```python
from build123d import *

# Parameters (mm, degrees)
SKETCH_1_W          = 10
SKETCH_1_H          = 10
SKETCH_1_W_2        = 8
SKETCH_1_H_2        = 8
EXTRUDE_1_DEPTH     = 40
SKETCH_2_R          = 1.6
CUT_EXTRUDE_1_DEPTH = 408.37168574
SKETCH_3_R          = 1.6
CUT_EXTRUDE_2_DEPTH = 10


with BuildPart() as part:
    # ｽｹｯﾁ1 → ﾎﾞｽ - 押し出し1 (new body)
    with BuildSketch(Plane.XY):
        Rectangle(SKETCH_1_W, SKETCH_1_H)
        Rectangle(SKETCH_1_W_2, SKETCH_1_H_2, mode=Mode.SUBTRACT)
    extrude(amount=EXTRUDE_1_DEPTH)

    # ｽｹｯﾁ2 → ｶｯﾄ - 押し出し1 (cut)
    with BuildSketch(Plane(origin=(0, 5, 0), x_dir=(1, 0, 0), z_dir=(0, 1, 0))):
        with Locations(Location((0, -5, 0), (0, 0, 270))):
            Circle(SKETCH_2_R)
        with Locations(Location((0, -35, 0), (0, 0, 270))):
            Circle(SKETCH_2_R)
    extrude(amount=-CUT_EXTRUDE_1_DEPTH, mode=Mode.SUBTRACT)

    # ｽｹｯﾁ3 → ｶｯﾄ - 押し出し2 (cut)
    with BuildSketch(Plane(origin=(5, 0, 0), x_dir=(0, 0, -1), z_dir=(1, 0, 0))):
        with Locations(Location((-20, 0, 0), (0, 0, 90))):
            Circle(SKETCH_3_R)
    extrude(amount=-CUT_EXTRUDE_2_DEPTH, mode=Mode.SUBTRACT)


solid = part.part
```
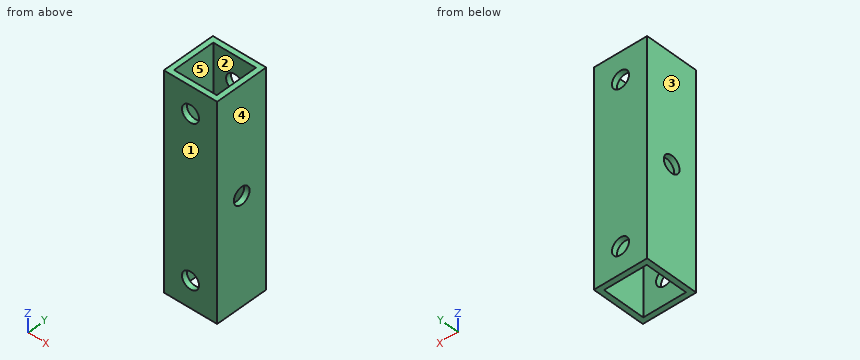
Model file for the job. Use its own axes, mm. Face numbers are marked on the shaded views. A direction names the side the tool comes from. Coordinates: 2 decimals unless noted, no trailing zeros. Loops run counter-clockwise (first coordinate to the right, second up) from the corner with the lowest first, then second, coordinate; pieces in that order, holes last. Notation, with made-up numbers: (0, 46.25) -> (41, 46.25) arc R19 cw to (41, 65.25) -> close; hole circle Ø5 at (81.25, -31.5). An arc over 180 degrees is marked (long way). Answer as a JSON object with one key per item and string values.
Q1. 3-axis set-ups, long thin cutter, end or side, ignore diameter. For the marked faces 1 and 2: which of +Z, -Z, +X, -X, +Y, -Y reach the whole face in a straight line?
Report:
{"face 1": "+Z, -Z, +X, -X, -Y", "face 2": "+Z, -Z"}
Q2. Cut at B-B (z = 35). List the corners of the cut face in (x, y).
Report:
{"outline": "(-5, -5) -> (-1.6, -5) -> (-1.6, -4) -> (-4, -4) -> (-4, 4) -> (-1.6, 4) -> (-1.6, 5) -> (-5, 5) -> close; (1.6, -5) -> (5, -5) -> (5, 5) -> (1.6, 5) -> (1.6, 4) -> (4, 4) -> (4, -4) -> (1.6, -4) -> close"}
Q3. Flat gauge pin, fed straight in: P1, Ø5, axis at x = 0.5, y = -2.5, coming from the +Z side. Where does the tip first touch, or does it go through?
Report:
{"P1": "stops at z = 40"}
Q4. Cut at C-C (y = -3). List the corners of the cut face in (x, z).
Report:
{"outline": "(-5, 0) -> (-4, 0) -> (-4, 40) -> (-5, 40) -> close; (4, 0) -> (5, 0) -> (5, 40) -> (4, 40) -> close"}
Q5. Pull direction X, two halves, no side cores. Call the marked faces 3, 4 and 5: released by +X, released by -X, zero draft, split by the parting line, or undercut.
Report:
{"face 3": "released by -X", "face 4": "released by +X", "face 5": "undercut"}
Q6. Cut at A-A (x = 0). List the corners of the cut face in (y, z).
Report:
{"outline": "(-5, 0) -> (-4, 0) -> (-4, 3.4) -> (-5, 3.4) -> close; (-5, 6.6) -> (-4, 6.6) -> (-4, 33.4) -> (-5, 33.4) -> close; (-5, 36.6) -> (-4, 36.6) -> (-4, 40) -> (-5, 40) -> close; (4, 0) -> (5, 0) -> (5, 3.4) -> (4, 3.4) -> close; (4, 6.6) -> (5, 6.6) -> (5, 33.4) -> (4, 33.4) -> close; (4, 36.6) -> (5, 36.6) -> (5, 40) -> (4, 40) -> close"}
Q7. Probe probe 1 along X at (y, z) = (-3.5, 24.5); probe 2 along Z at (x, y) = (4.55, 0). List the from-to ranges inside material, lowest first.
Report:
{"probe 1": "x = -5 to -4, 4 to 5", "probe 2": "z = 0 to 18.4, 21.6 to 40"}
